The listing builds one solid part. Answer for the finished solid, in the listing's coordinates (mm). Give positions to 0.01 mm unless a question says otherwise; leave off trailing zeros. Write each loop counter-clockwise with the first axis right and the second up, starting at its lowest first coordinate (ties: lowest second). Pieces come first, ordered by that corner, then holes.
Autodesk Inventor part; units mm, degrees
ref_plane "YZ Plane" through (0, 0, 0) normal (1, 0, 0) x (0, 1, 0)
ref_plane "XZ Plane" through (0, 0, 0) normal (0, 1, 0) x (-1, 0, 0)
ref_plane "XY Plane" through (0, 0, 0) normal (0, 0, 1) x (1, 0, 0)
sketch "Boceto1" plane through (0, 0, 0) normal (0, 1, 0) x (-1, 0, 0)
  line L0 (10, 0) -> (10, -40)
  line L1 (10, -40) -> (-10, -40)
  line L2 (-10, -40) -> (-10, 40)
  line L3 (-10, 40) -> (10, 40)
  line L4 (10, 40) -> (10, 0)
  line L5 (0, 0) -> (0, 20)
  line L6 (0, 20) -> (5, 20)
  line L7 (0, 0) -> (0, -20)
  line L8 (0, -20) -> (5, -20)
  line L9 (0, 20) -> (-5, 20)
  line L10 (0, -20) -> (-5, -20)
  circle A0 centre (5, 20) radius 2
  circle A1 centre (5, -20) radius 2
  circle A2 centre (-5, -20) radius 2
  circle A3 centre (-5, 20) radius 2
  dimension "d1" = 40
  dimension "d2" = 20
  dimension "d3" = 80
  dimension "d5" = 20
  dimension "d6" = 5
  dimension "d7" = 20
  dimension "d8" = 5
  dimension "d9" = 5
  dimension "d10" = 4
  dimension "d11" = 4
  dimension "d12" = 4
  dimension "d13" = 4
extrude "Extrusión1" add sketch "Boceto1" along normal blind 3
equation "\"Radio_pliegue\" = Grosor"
equation "\"Anchura_desahogo_plegado\" = Grosor"
equation "\"Profundidad_desahogo_plegado\" = 0.5 * Grosor"
equation "\"Tamaño_destalonado\" = 4 * Grosor"
equation "\"Remanente_mínimo\" = 2 * Grosor"
equation "\"Radiodetransición\" = Radio_pliegue"
equation "\"Tamaño_de_radio_de_Jacobi\" = Radio_pliegue"
equation "\"TamañoSeparación\" = Grosor"
properties part number "Soporte_Techo"
Item 1: Consider probe 1 along Z at (x, y) = (5, 2.3); probe 2 along Z at (x, y) = (-3.75, 2.45). Determine where each line is inside the solid, lowest interval first.
Conclusion:
probe 1: z = -40 to -22, -18 to 18, 22 to 40
probe 2: z = -40 to -21.56, -18.44 to 18.44, 21.56 to 40
Item 2: A cutting plane is placed at A-A, the plane x = 5. Give the vertices of the cut face in (y, z), plus the area to 3 significant figures.
Conclusion:
outline: (0, -40) - (3, -40) - (3, -22) - (0, -22) - close; (0, -18) - (3, -18) - (3, 18) - (0, 18) - close; (0, 22) - (3, 22) - (3, 40) - (0, 40) - close
area: 216 mm2
Item 3: A cutting plane is placed at C-C, the plane z = -20. Give the vertices of the cut face in (x, y).
Conclusion:
outline: (-10, 0) - (-7, 0) - (-7, 3) - (-10, 3) - close; (-3, 0) - (3, 0) - (3, 3) - (-3, 3) - close; (7, 0) - (10, 0) - (10, 3) - (7, 3) - close
Item 4: A cutting plane is placed at B-B, the plane y = 2.5. Give the vertices of the cut face in (x, z).
Conclusion:
outline: (-10, -40) - (10, -40) - (10, 40) - (-10, 40) - close; hole circle Ø4 at (-5, -20); hole circle Ø4 at (-5, 20); hole circle Ø4 at (5, -20); hole circle Ø4 at (5, 20)
